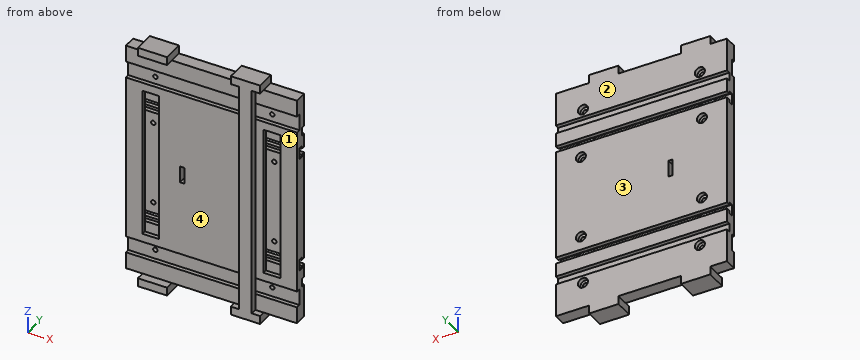
Autodesk Inventor part; units mm, degrees
ref_plane "YZ Plane" through (0, 0, 0) normal (1, 0, 0) x (0, 1, 0)
ref_plane "XZ Plane" through (0, 0, 0) normal (0, 1, 0) x (-1, 0, 0)
sketch "Sketch3" plane through (0, 0, 0) normal (0, 0, 1) x (1, 0, 0)
  line L0 (0, -9.525) -> (9.525, -9.525)
  line L1 (9.525, -9.525) -> (9.525, 0)
  line L2 (0, 0) -> (0, -9.525) construction
  line L3 (0, 0) -> (9.525, 0) construction
  line L4 (0, -9.525) -> (-9.525, -9.525)
  line L5 (-9.525, -9.525) -> (-9.525, 0)
  line L6 (9.525, 0) -> (73.025, 0)
  line L7 (-187.325, 0) -> (-187.325, 19.05)
  line L8 (-187.325, 0) -> (-9.525, 0)
  line L9 (73.025, 0) -> (73.025, 19.05)
  line L10 (73.025, 19.05) -> (-187.325, 19.05)
  dimension "d0" = 9.525
  dimension "d1" = 9.525
  dimension "d6" = 63.5
  dimension "d8" = 19.05
  dimension "d9" = 177.8
extrude "Extrusion1" add sketch "Sketch3" along normal mid plane 355.6
sketch "Sketch4" plane through (0, 0, 177.8) normal (0, 0, 1) x (1, 0, 0)
  line L0 (-187.325, 19.05) -> (73.025, 19.05) construction
  line L1 (0, 19.05) -> (0, -9.525) construction
  line L2 (9.525, -9.525) -> (-9.525, -9.525) construction
  line L3 (0, -9.525) -> (-22.225, -9.525)
  line L4 (-22.225, -9.525) -> (-22.225, 19.05)
  line L5 (-22.225, 19.05) -> (0, 19.05)
  line L6 (187.325, 19.05) -> (-73.025, 19.05) construction
  line L7 (0, -9.525) -> (22.225, -9.525)
  line L8 (22.225, -9.525) -> (22.225, 19.05)
  line L9 (0, 19.05) -> (22.225, 19.05)
  point P0 (0, 0)
  dimension "d12" = 22.225
extrude "Extrusion2" add sketch "Sketch4" along normal blind 12.7
mirror "Mirror1" about plane through (0, 0, 0) normal (0, 0, 1) of "Extrusion2"
sketch "Sketch6" plane through (-187.325, 0, -177.8) normal (0, -1, 0) x (1, 0, 0)
  line L0 (82.55, 165.1) -> (88.9, 165.1)
  line L1 (88.9, 165.1) -> (88.9, 190.5)
  line L2 (88.9, 190.5) -> (82.55, 190.5)
  line L3 (82.55, 190.5) -> (82.55, 165.1)
  line L4 (82.55, 165.1) -> (88.9, 190.5) construction
  line L5 (88.9, 165.1) -> (82.55, 190.5) construction
  line L6 (177.8, 0) -> (177.8, 355.6)
  point P0 (187.325, 177.8)
  point P1 (85.725, 177.8)
  dimension "d16" = 12.7
  dimension "d18" = 6.35
  dimension "d19" = 88.9
extrude "Extrusion3" cut sketch "Sketch6" against normal through all
sketch "Sketch7" plane through (0, 0, 177.8) normal (0, 0, 1) x (1, 0, 0)
  line L0 (-187.325, 19.05) -> (-22.225, 19.05)
  line L1 (-161.925, 19.05) -> (-117.475, 19.05)
  line L2 (-117.475, 19.05) -> (-117.475, -12.7)
  line L3 (-117.475, -12.7) -> (-161.925, -12.7)
  line L4 (-161.925, -12.7) -> (-161.925, 19.05)
  line L5 (-187.325, 19.05) -> (-187.325, 0)
  point P0 (0, 0)
  dimension "d22" = 44.45
  dimension "d23" = 31.75
  dimension "d24" = 25.4
extrude "Extrusion4" add sketch "Sketch7" along normal blind 12.7
mirror "Mirror2" about plane through (0, 0, 0) normal (0, 0, 1) of "Extrusion4"
sketch "Sketch9" plane through (73.025, 0, 177.8) normal (1, 0, 0) x (0, 0, -1)
  line L0 (355.6, 19.05) -> (0, 19.05)
  line L1 (50.8, 19.05) -> (63.5, 19.05)
  line L2 (63.5, 19.05) -> (63.5, 12.7)
  line L3 (63.5, 12.7) -> (50.8, 12.7)
  line L4 (50.8, 12.7) -> (50.8, 19.05)
  line L5 (0, 0) -> (0, 19.05)
  point P0 (177.8, 0)
  dimension "d28" = 12.7
  dimension "d29" = 6.35
  dimension "d30" = 50.8
extrude "Extrusion5" cut sketch "Sketch9" against normal through all
mirror "Mirror3" about plane through (0, 0, 0) normal (0, 0, 1) of "Extrusion5"
sketch "Sketch12" plane through (73.025, 0, 177.8) normal (1, 0, 0) x (0, 0, -1)
  line L0 (355.6, 0) -> (0, 0) construction
  line L1 (88.9, 0) -> (88.9, 16.5009) construction
  line L2 (0, 0) -> (0, 19.05)
  line L3 (50.8, 19.05) -> (0, 19.05)
  line L4 (84.1375, 19.05) -> (84.1375, 12.7)
  line L5 (84.1375, 12.7) -> (80.1624, 12.7)
  line L6 (80.1624, 12.7) -> (80.1624, 6.35)
  line L7 (80.1624, 6.35) -> (88.9, 6.35)
  line L8 (93.6625, 19.05) -> (93.6625, 12.7)
  line L9 (93.6625, 12.7) -> (97.6376, 12.7)
  line L10 (97.6376, 12.7) -> (97.6376, 6.35)
  line L11 (97.6376, 6.35) -> (88.9, 6.35)
  line L12 (84.1375, 19.05) -> (93.6625, 19.05)
  point P0 (177.8, 0)
  dimension "d46" = 88.9
  dimension "d47" = 4.7625
  dimension "d48" = 6.35
  dimension "d49" = 6.35
  dimension "d50" = 8.7376
extrude "Extrusion8" cut sketch "Sketch12" against normal through all
mirror "Mirror4" about plane through (0, 0, 0) normal (0, 0, 1) of "Extrusion8"
ref_plane "Work Plane1" through (-57.15, 0, 177.8) normal (1, 0, 0) x (0, 0, -1)
sketch "Sketch13" plane through (-57.15, 0, 177.8) normal (1, 0, 0) x (0, 0, -1)
  line L0 (25.4, 0) -> (50.8, 0)
  line L1 (50.8, 0) -> (50.8, 6.35)
  line L2 (50.8, 6.35) -> (25.4, 6.35)
  line L3 (25.4, 6.35) -> (25.4, 0)
  line L4 (0, 0) -> (0, 19.05)
  point P0 (177.8, 0)
  dimension "d54" = 25.4
  dimension "d55" = 6.35
  dimension "d56" = 25.4
extrude "Extrusion9" cut sketch "Sketch13" along normal mid plane 260.35
mirror "Mirror5" about plane through (0, 0, 0) normal (0, 0, 1) of "Extrusion9"
sketch "Sketch14" plane through (0, 0, 0) normal (0, 0, 1) x (1, 0, 0)
  line L0 (-187.325, 0) -> (-161.925, 0)
  line L1 (-161.925, 0) -> (-136.525, 0)
  line L2 (-136.525, 0) -> (-136.525, 6.35)
  line L3 (-136.525, 6.35) -> (-161.925, 6.35)
  line L4 (-161.925, 6.35) -> (-161.925, 0)
  line L5 (-187.325, 19.05) -> (-187.325, 0)
  point P0 (0, 0)
  dimension "d59" = 25.4
  dimension "d60" = 6.35
  dimension "d61" = 25.4
extrude "Extrusion10" cut sketch "Sketch14" along normal mid plane 228.6
mirror "Mirror6" about plane through (-57.15, 0, 177.8) normal (1, 0, 0) of "Extrusion10"
sketch "Sketch16" plane through (-161.925, 6.35, -80.1624) normal (0, -1, 0) x (1, 0, 0)
  circle A0 centre (12.7, 143.6624) radius 3.3782
  line L0 (0, 194.4624) -> (25.4, 194.4624)
  line L1 (0, -34.1376) -> (0, 194.4624)
  point P0 (161.925, 80.1624)
  dimension "d71" = 6.7564
  dimension "d72" = 50.8
  dimension "d73" = 12.7
extrude "Extrusion11" cut sketch "Sketch16" against normal through all
sketch "Sketch17" plane through (-187.325, 19.05, 84.1375) normal (0, 1, 0) x (1, 0, 0)
  circle A0 centre (38.1, 20.6375) radius 3.3782
  circle A1 centre (38.1, 20.6375) radius 7.62
  point P0 (187.325, 84.1375)
  dimension "d76" = 15.24
extrude "Extrusion12" cut sketch "Sketch17" against normal blind 6.35
mirror "Mirror7" about plane through (0, 0, 0) normal (0, 0, 1) of "Extrusion12", "Extrusion11"
mirror "Mirror8" about plane through (-57.15, 0, 177.8) normal (1, 0, 0) of "Extrusion12", "Extrusion11", "Mirror7"
sketch "Sketch18" plane through (-171.45, 6.35, 152.4) normal (0, -1, 0) x (1, 0, 0)
  circle A0 centre (203.2, -14.094) radius 3.3782
  line L0 (228.6, 0) -> (228.6, -25.4)
  point P0 (171.45, -152.4)
  dimension "d79" = 6.7564
  dimension "d80" = 25.4
extrude "Extrusion13" cut sketch "Sketch18" against normal through all
sketch "Sketch19" plane through (22.225, 19.05, 177.8) normal (0, 1, 0) x (1, 0, 0)
  circle A0 centre (9.525, 39.494) radius 3.3782
  circle A1 centre (9.525, 39.494) radius 7.62
  point P0 (-22.225, 177.8)
  dimension "d83" = 15.24
extrude "Extrusion14" cut sketch "Sketch19" against normal blind 6.35
mirror "Mirror9" about plane through (-57.15, 0, 177.8) normal (1, 0, 0) of "Extrusion13", "Extrusion14"
mirror "Mirror10" about plane through (0, 0, 0) normal (0, 0, 1) of "Extrusion14", "Extrusion13", "Mirror9"
equation "\"d10\" = length"
equation "\"width\" = 260.35"
equation "\"length\" = 355.6"
equation "\"d53\" = -0.5 * width"
properties part number "BandSawJigBottom" material "LCP Plastic"
The model under review builds one solid part; all positions refer to its coordinate system, in mm. Face numbers are marked on the shaded views. A direction names the side the tool comes from. Give positions to 0.01 mm unless a question says otherwise; leave off trailing zeros. Loops run counter-clockwise (first coordinate to the right, second up) from the corner with the lowest first, then second, coordinate; pieces in that order, holes last. Notation, with made-up numbers: (0, -24.5) - (42, -24.5) arc R22 cw to (42, -1.5) - close; hole circle Ø10 at (74, 15.5). An arc over 180 degrees is marked (long way). Answer as a JSON object with one key per item and string values.
Q1. Mouldability with a two-part tool opening along Z and no side actions: class the marked faces 1 and 2 as +Z half, -Z half, draft (parallel to the pull), parting line (faces both ways), or undercut.
Worked out:
{"face 1": "undercut", "face 2": "draft"}
Q2. Add section A-A on y = -5.5. State the section outline as (x, z) points (3 decimals), plus the area to 3 significant figures.
Worked out:
{"outline": "(-161.925, -190.5) - (-117.475, -190.5) - (-117.475, -177.8) - (-161.925, -177.8) - close; (-161.925, 177.8) - (-117.475, 177.8) - (-117.475, 190.5) - (-161.925, 190.5) - close; (-22.225, -190.5) - (22.225, -190.5) - (22.225, -177.8) - (9.525, -177.8) - (9.525, 177.8) - (22.225, 177.8) - (22.225, 190.5) - (-22.225, 190.5) - (-22.225, 177.8) - (-9.525, 177.8) - (-9.525, -177.8) - (-22.225, -177.8) - close", "area": "9,030 mm^2"}
Q3. Add section B-B on z = 39.5. State the section outline as (x, y) points (3 decimals).
Worked out:
{"outline": "(-187.325, 0) - (-161.925, 0) - (-161.925, 6.35) - (-136.525, 6.35) - (-136.525, 0) - (-9.525, 0) - (-9.525, -9.525) - (9.525, -9.525) - (9.525, 0) - (22.225, 0) - (22.225, 6.35) - (47.625, 6.35) - (47.625, 0) - (73.025, 0) - (73.025, 19.05) - (-187.325, 19.05) - close"}
Q4. Insertion check: pin 1 (12.5 mm diameter, centred on x = -155, z = 1, fed in from -Y); pin 2 (14 mm diameter, centred on x = -179.5, z = -91.5, fed in from +Y); pin 3 (2 mm diameter, centred on x = -23.5, z = -8.5, fed in from -Y); pin 4 (4 mm diameter, centred on x = -75, y = 10, fed in from +Z). Each pin has a flat end and moves straight along its axis. Give the tip position at first contact, or say it passes through.
Worked out:
{"pin 1": "stops at y = 6.35", "pin 2": "stops at y = 19.05", "pin 3": "stops at y = 0", "pin 4": "stops at z = 177.8"}
Q5. For the marked faces 3 and 4, list the 3-axis set-ups (+Z, -Z, +X, -X, +Y, -Y) from which the entire face can be reached by the end or side of a thin tool; tool diameter is ignored.
Worked out:
{"face 3": "+Z, -Z, +X, -X, +Y", "face 4": "-X, -Y"}
Q6. To check wall thickness, follow line 1 along Z through (x, y) = (-82, 2); line 2 along Z through (x, y) = (-137.5, 10); line 3 along X through (y, z) = (1.5, 45) (3 decimals). State the ranges of each line that lie inside material, in increasing order.
Worked out:
{"line 1": "z = -177.8 to -152.4, -127 to 127, 152.4 to 177.8", "line 2": "z = -190.5 to -97.64, -80.16 to 80.16, 97.64 to 190.5", "line 3": "x = -187.325 to -161.925, -136.525 to 22.225, 47.625 to 73.025"}
